from build123d import *

# Parameters (mm, degrees)
SKETCH1_R           = 3.7
SKETCH1_R_2         = 1.6
SKETCH1_R_3         = 2.6
SKETCH1_W           = 110
SKETCH1_H           = 70
BOSS_EXTRUDE1_DEPTH = 3.175
FILLET1_R           = 10
CUT_EXTRUDE1_DEPTH  = 3.175
SKETCH3_3_R         = 1.6
BOSS_EXTRUDE2_DEPTH = 3.175
SKETCH4_R           = 1.6
BOSS_EXTRUDE3_DEPTH = 3.175
FILLET2_R           = 5


with BuildPart() as part:
    # Sketch1 → Boss-Extrude1 (new body)
    with BuildSketch(Plane(origin=(0, 0, 0), x_dir=(1, 0, 0), z_dir=(0, 1, 0))):
        with BuildLine():
            Line((-114.5, 114.5), (-114.5, 95.706582846))
            ThreePointArc((-114.5, 95.706582846), (-80, 0), (-114.5, -95.706582846))
            Line((-114.5, -95.706582846), (-114.5, -114.5))
            Line((-114.5, -114.5), (-89.049143735, -114.5))
            ThreePointArc((-89.049143735, -114.5), (-58.383323853, -78.812639556), (-14.791551643, -61.1))
            ThreePointArc((-14.791551643, -61.1), (0, -65), (14.791551643, -61.1))
            ThreePointArc((14.791551643, -61.1), (58.383323853, -78.812639556), (89.049143735, -114.5))
            Line((89.049143735, -114.5), (114.5, -114.5))
            Line((114.5, -114.5), (114.5, -95.706582846))
            ThreePointArc((114.5, -95.706582846), (80, 0), (114.5, 95.706582846))
            Line((114.5, 95.706582846), (114.5, 114.5))
            Line((114.5, 114.5), (89.049143735, 114.5))
            ThreePointArc((89.049143735, 114.5), (58.383323853, 78.812639556), (14.791551643, 61.1))
            ThreePointArc((14.791551643, 61.1), (0, 65), (-14.791551643, 61.1))
            ThreePointArc((-14.791551643, 61.1), (-58.383323853, 78.812639556), (-89.049143735, 114.5))
            Line((-89.049143735, 114.5), (-114.5, 114.5))
        make_face()
        with Locations((77.9, 55)):
            Circle(SKETCH1_R, mode=Mode.SUBTRACT)
        with Locations((-10, 50)):
            Circle(SKETCH1_R_2, mode=Mode.SUBTRACT)
        with Locations((-104.5, 104.5)):
            Circle(SKETCH1_R_2, mode=Mode.SUBTRACT)
        with Locations((-5, 60)):
            Circle(SKETCH1_R_2, mode=Mode.SUBTRACT)
        with Locations((77.9, -55)):
            Circle(SKETCH1_R, mode=Mode.SUBTRACT)
        with Locations((-77.9, 55)):
            Circle(SKETCH1_R_3, mode=Mode.SUBTRACT)
        with Locations((-104.5, -104.5)):
            Circle(SKETCH1_R_2, mode=Mode.SUBTRACT)
        with Locations((-77.9, -55)):
            Circle(SKETCH1_R_3, mode=Mode.SUBTRACT)
        with Locations((-10, -50)):
            Circle(SKETCH1_R_2, mode=Mode.SUBTRACT)
        with Locations((-5, -60)):
            Circle(SKETCH1_R_2, mode=Mode.SUBTRACT)
        with Locations((104.5, -104.5)):
            Circle(SKETCH1_R_2, mode=Mode.SUBTRACT)
        with Locations((5, -60)):
            Circle(SKETCH1_R_2, mode=Mode.SUBTRACT)
        with Locations((10, -50)):
            Circle(SKETCH1_R_2, mode=Mode.SUBTRACT)
        with Locations((104.5, 104.5)):
            Circle(SKETCH1_R_2, mode=Mode.SUBTRACT)
        with Locations((10, 50)):
            Circle(SKETCH1_R_2, mode=Mode.SUBTRACT)
        with Locations((5, 60)):
            Circle(SKETCH1_R_2, mode=Mode.SUBTRACT)
        Rectangle(SKETCH1_W, SKETCH1_H, mode=Mode.SUBTRACT)
    extrude(amount=BOSS_EXTRUDE1_DEPTH)

    # Fillet1
    fillet1_edges = [part.edges().sort_by_distance(p)[0] for p in [
        (-114.5, 1.5875, 114.5),
        (-114.5, 1.5875, 95.706582846),
        (-114.5, 1.5875, -95.706582846),
        (-114.5, 1.5875, -114.5),
        (-89.049143735, 1.5875, -114.5),
        (-14.791551643, 1.5875, -61.1),
        (14.791551643, 1.5875, -61.1),
        (89.049143735, 1.5875, -114.5),
        (114.5, 1.5875, -114.5),
        (114.5, 1.5875, -95.706582846),
        (114.5, 1.5875, 95.706582846),
        (114.5, 1.5875, 114.5),
        (89.049143735, 1.5875, 114.5),
        (14.791551643, 1.5875, 61.1),
        (-14.791551643, 1.5875, 61.1),
        (-89.049143735, 1.5875, 114.5),
        (-55, 1.5875, -35),
        (-55, 1.5875, 35),
        (55, 1.5875, 35),
        (55, 1.5875, -35),
    ]]
    fillet(fillet1_edges, radius=FILLET1_R)

    # Sketch3 → Cut-Extrude1 (cut)
    with BuildSketch(Plane(origin=(0, 3.175, 0), x_dir=(1, 0, 0), z_dir=(0, 1, 0))):
        with BuildLine():
            Line((-86.338513092, -109.545454545), (86.338513092, -109.545454545))
            ThreePointArc((86.338513092, -109.545454545), (57.482053735, -78.172049406), (18.181186858, -61.666666667))
            ThreePointArc((18.181186858, -61.666666667), (-41.646726907, -69.084928983), (-86.338513092, -109.545454545))
        make_face()
        with BuildLine():
            Line((-86.338513092, 109.545454545), (86.338513092, 109.545454545))
            ThreePointArc((86.338513092, 109.545454545), (57.482053735, 78.172049406), (18.181186858, 61.666666667))
            ThreePointArc((18.181186858, 61.666666667), (-41.646726907, 69.084928983), (-86.338513092, 109.545454545))
        make_face()
    extrude(amount=-CUT_EXTRUDE1_DEPTH, mode=Mode.SUBTRACT)

    # Sketch3<3> → Boss-Extrude2 (add)
    with BuildSketch(Plane(origin=(0, 3.175, 0), x_dir=(1, 0, 0), z_dir=(0, 1, 0))):
        with BuildLine():
            ThreePointArc((-3.401046245, -60.057852312), (-5.079900187, -58.401996258), (-6.585208119, -60.217060406))
            ThreePointArc((-6.585208119, -60.217060406), (-4.993761694, -60.124766112), (-3.401046245, -60.057852312))
        make_face()
        with BuildLine():
            ThreePointArc((3.401046245, -60.057852312), (4.993761694, -60.124766112), (6.585208119, -60.217060406))
            ThreePointArc((6.585208119, -60.217060406), (5.079900187, -58.401996258), (3.401046245, -60.057852312))
        make_face()
        with BuildLine():
            ThreePointArc((-3.401046245, 60.057852312), (-4.993761694, 60.124766112), (-6.585208119, 60.217060406))
            ThreePointArc((-6.585208119, 60.217060406), (-5.079900187, 58.401996258), (-3.401046245, 60.057852312))
        make_face()
        with BuildLine():
            ThreePointArc((3.401046245, 60.057852312), (5.079900187, 58.401996258), (6.585208119, 60.217060406))
            ThreePointArc((6.585208119, 60.217060406), (4.993761694, 60.124766112), (3.401046245, 60.057852312))
        make_face()
        with Locations((10, 50)):
            Circle(SKETCH3_3_R)
        with Locations((-10, 50)):
            Circle(SKETCH3_3_R)
        with Locations((-10, -50)):
            Circle(SKETCH3_3_R)
        with Locations((10, -50)):
            Circle(SKETCH3_3_R)
    extrude(amount=-BOSS_EXTRUDE2_DEPTH)

    # Sketch4 → Boss-Extrude3 (add)
    with BuildSketch(Plane(origin=(0, 3.175, 0), x_dir=(1, 0, 0), z_dir=(0, 1, 0))):
        with BuildLine():
            Line((-24.5, -15), (-24.5, 15))
            Line((-24.5, 15), (-45, 35))
            ThreePointArc((-45, 35), (-52.071067812, 32.071067812), (-55, 25))
            Line((-55, 25), (-55, -25))
            ThreePointArc((-55, -25), (-52.071067812, -32.071067812), (-45, -35))
            Line((-45, -35), (-24.5, -15))
        make_face()
        with Locations((-28.5, 10)):
            Circle(SKETCH4_R, mode=Mode.SUBTRACT)
        with Locations((-28.5, -10)):
            Circle(SKETCH4_R, mode=Mode.SUBTRACT)
        with Locations((-41.5, 0)):
            Circle(SKETCH4_R, mode=Mode.SUBTRACT)
    extrude(amount=-BOSS_EXTRUDE3_DEPTH)

    # Fillet2
    fillet2_edges = [part.edges().sort_by_distance(p)[0] for p in [
        (-45, 1.5875, 35),
        (-45, 1.5875, -35),
    ]]
    fillet(fillet2_edges, radius=FILLET2_R)


solid = part.part
For this review, take the finished solid that the model builds, in its own axes (mm). A direction names the side the tool comes from. Coordinates: 2 decimals unless noted, no trailing zeros. Order: outer loops, then holes, each group sorted by start corner. A loop starts at its lowest first (then second) coordinate and runs counter-clockwise, first axis right, second up. Notation, with made-up numbers: (56, 12.25) - (93, 12.25) arc R33 cw to (93, 47.25) - close; hole circle Ø9 at (-19, 71). An arc over 180 degrees is marked (long way). Answer as CSV lines item,"result". Start each with the question number.
1) To check wall thickness, follow line 1 along X through (y, z) = (1.55, 10); line 2 along X through (y, z) = (1.5, -104.5); line 3 along Z through (x, y) = (104.5, 0.7). State the ranges of each line that lie inside material, in increasing order. Write a range as [from, to].
2) Draft analysis for pull direction Z (two halves, no side actions). For faces 5 (the cylindrical face through (111.49, 1.61, 111.65)), 6 (the cylindrical face through (89.932, 1.61, -113.137)), 7 (the flat face through (-30.27, 1.61, -20.63)), 8 (the flat face through (-27, 0, -2)), state which applies: +Z half, -Z half, draft (parallel to the pull), parting line (faces both ways), or undercut.
3) Add section A-A (x = 39.5). State the section outline as (y, z) points (3 decimals), then the cut area to 3 significant figures.
4) Machinability: for faces 1 (the cylindrical face through (52.15, 1.61, -31.99)), 2 (the cylindrical face through (-90.06, 1.61, -113.21)), 3 (the cylindrical face through (80.007, 1.565, 1.405)), 4 (the cylindrical face through (89.932, 1.61, 113.137)), which of the approach directions +Z, -Z, +X, -X, +Y, -Y give a long, thin tool a straight path to every point of the face, cutting with its end or side? Answer none if there is none.
5) Add section B-B (z = -55). State the section outline as (x, y) points (3 decimals), then the cut area to 3 significant figures.
6) Add section C-C (y = 1.4). Count the separate pieces of the cut face and the enclosed holes in it, then the cut area to 3 significant figures.
7) Insertion check: P1, Ø1.5, axis at x = 22, y = 0.5, coming from the -Z side; P2, Ø1, axis at x = 15, y = 2, coming from the +Z side; P3, Ø1.6, axis at x = 7, y = 2, coming from the -Z side. Each pin has a flat end and moves straight along its axis. Give the tip position at first contact, or say it passes through.
Result:
1,line 1,"[-80.33, -30.1], [-26.9, -24.5], [55, 80.33]"
1,line 2,"[-114.5, -106.1], [-102.9, -83.19], [83.19, 102.9], [106.1, 114.5]"
1,line 3,"[-114.5, -106.1], [-102.9, -82.16], [82.16, 102.9], [106.1, 114.5]"
2,face 5,"+Z half"
2,face 6,"-Z half"
2,face 7,"undercut"
2,face 8,"draft"
3,outline,"(0, -68.132) - (3.175, -68.132) - (3.175, -35) - (0, -35) - close; (0, 35) - (3.175, 35) - (3.175, 68.132) - (0, 68.132) - close"
3,area,"210 mm^2"
4,face 1,"+Y, -Y"
4,face 2,"-Z, +Y, -Y"
4,face 3,"+X, +Y, -Y"
4,face 4,"+Z, +Y, -Y"
5,outline,"(-90.447, 0) - (-80.5, 0) - (-80.5, 3.175) - (-90.447, 3.175) - close; (-75.3, 0) - (74.2, 0) - (74.2, 3.175) - (-75.3, 3.175) - close; (81.6, 0) - (90.447, 0) - (90.447, 3.175) - (81.6, 3.175) - close"
5,area,"534 mm^2"
6,separate pieces,"1"
6,enclosed holes,"12"
6,area,"23,400 mm^2"
7,P1,"z = -62.62"
7,P2,"z = 61.21"
7,P3,"z = -60.3"
